Part model, mm, in its own coordinate system. Give positions to 0.01 mm unless a question says otherwise; leave off trailing zeros. Write each loop counter-clockwise with the first axis right and the second up, starting at its lowest first coordinate (ties: lowest second). Pieces come first, ordered by that corner, then holes.
from build123d import *

# Parameters (mm, degrees)
SKETCH_1_R      = 2
SKETCH_1_R_2    = 3.5
SKETCH_1_R_3    = 1
EXTRUDE_2_DEPTH = 0.5


with BuildPart() as part:
    # Эскиз1 → Бобышка-Вытянуть2 (new body)
    with BuildSketch(Plane(origin=(0, 0, 0), x_dir=(1, 0, 0), z_dir=(0, 1, 0))):
        with BuildLine():
            Line((-100, 38.5), (100, 38.5))
            ThreePointArc((100, 38.5), (100.707106781, 38.207106781), (101, 37.5))
            Line((101, 37.5), (101, -37.5))
            ThreePointArc((101, -37.5), (100.707106781, -38.207106781), (100, -38.5))
            Line((100, -38.5), (-100, -38.5))
            ThreePointArc((-100, -38.5), (-100.707106781, -38.207106781), (-101, -37.5))
            Line((-101, -37.5), (-101, 37.5))
            ThreePointArc((-101, 37.5), (-100.707106781, 38.207106781), (-100, 38.5))
        make_face()
        with Locations(Location((-88, 29, 0), (0, 0, 270))):
            Circle(SKETCH_1_R, mode=Mode.SUBTRACT)
        with Locations(Location((88, 29, 0), (0, 0, 270))):
            Circle(SKETCH_1_R, mode=Mode.SUBTRACT)
        with Locations(Location((88, -29, 0), (0, 0, 270))):
            Circle(SKETCH_1_R, mode=Mode.SUBTRACT)
        with Locations(Location((-88, -29, 0), (0, 0, 270))):
            Circle(SKETCH_1_R, mode=Mode.SUBTRACT)
        with Locations(Location((92, -10, 0), (0, 0, 270))):
            Circle(SKETCH_1_R_2, mode=Mode.SUBTRACT)
        with Locations(Location((0, 3, 0), (0, 0, 270))):
            Circle(SKETCH_1_R_3, mode=Mode.SUBTRACT)
        with Locations(Location((0, 7, 0), (0, 0, 270))):
            Circle(SKETCH_1_R_3, mode=Mode.SUBTRACT)
        with Locations(Location((0, 11, 0), (0, 0, 270))):
            Circle(SKETCH_1_R_3, mode=Mode.SUBTRACT)
        with Locations(Location((0, 15, 0), (0, 0, 270))):
            Circle(SKETCH_1_R_3, mode=Mode.SUBTRACT)
        with Locations(Location((0, 19, 0), (0, 0, 270))):
            Circle(SKETCH_1_R_3, mode=Mode.SUBTRACT)
        with Locations(Location((2.598076211, 1.5, 0), (0, 0, 270))):
            Circle(SKETCH_1_R_3, mode=Mode.SUBTRACT)
        with Locations(Location((6.062177826, 3.5, 0), (0, 0, 270))):
            Circle(SKETCH_1_R_3, mode=Mode.SUBTRACT)
        with Locations(Location((9.526279442, 5.5, 0), (0, 0, 270))):
            Circle(SKETCH_1_R_3, mode=Mode.SUBTRACT)
        with Locations(Location((12.990381057, 7.5, 0), (0, 0, 270))):
            Circle(SKETCH_1_R_3, mode=Mode.SUBTRACT)
        with Locations(Location((16.454482672, 9.5, 0), (0, 0, 270))):
            Circle(SKETCH_1_R_3, mode=Mode.SUBTRACT)
        with Locations(Location((2.598076211, -1.5, 0), (0, 0, 270))):
            Circle(SKETCH_1_R_3, mode=Mode.SUBTRACT)
        with Locations(Location((6.062177826, -3.5, 0), (0, 0, 270))):
            Circle(SKETCH_1_R_3, mode=Mode.SUBTRACT)
        with Locations(Location((9.526279442, -5.5, 0), (0, 0, 270))):
            Circle(SKETCH_1_R_3, mode=Mode.SUBTRACT)
        with Locations(Location((12.990381057, -7.5, 0), (0, 0, 270))):
            Circle(SKETCH_1_R_3, mode=Mode.SUBTRACT)
        with Locations(Location((16.454482672, -9.5, 0), (0, 0, 270))):
            Circle(SKETCH_1_R_3, mode=Mode.SUBTRACT)
        with Locations(Location((0, -3, 0), (0, 0, 270))):
            Circle(SKETCH_1_R_3, mode=Mode.SUBTRACT)
        with Locations(Location((0, -7, 0), (0, 0, 270))):
            Circle(SKETCH_1_R_3, mode=Mode.SUBTRACT)
        with Locations(Location((0, -11, 0), (0, 0, 270))):
            Circle(SKETCH_1_R_3, mode=Mode.SUBTRACT)
        with Locations(Location((0, -15, 0), (0, 0, 270))):
            Circle(SKETCH_1_R_3, mode=Mode.SUBTRACT)
        with Locations(Location((0, -19, 0), (0, 0, 270))):
            Circle(SKETCH_1_R_3, mode=Mode.SUBTRACT)
        with Locations(Location((-2.598076211, -1.5, 0), (0, 0, 270))):
            Circle(SKETCH_1_R_3, mode=Mode.SUBTRACT)
        with Locations(Location((-6.062177826, -3.5, 0), (0, 0, 270))):
            Circle(SKETCH_1_R_3, mode=Mode.SUBTRACT)
        with Locations(Location((-9.526279442, -5.5, 0), (0, 0, 270))):
            Circle(SKETCH_1_R_3, mode=Mode.SUBTRACT)
        with Locations(Location((-12.990381057, -7.5, 0), (0, 0, 270))):
            Circle(SKETCH_1_R_3, mode=Mode.SUBTRACT)
        with Locations(Location((-16.454482672, -9.5, 0), (0, 0, 270))):
            Circle(SKETCH_1_R_3, mode=Mode.SUBTRACT)
        with Locations(Location((-2.598076211, 1.5, 0), (0, 0, 270))):
            Circle(SKETCH_1_R_3, mode=Mode.SUBTRACT)
        with Locations(Location((-6.062177826, 3.5, 0), (0, 0, 270))):
            Circle(SKETCH_1_R_3, mode=Mode.SUBTRACT)
        with Locations(Location((-9.526279442, 5.5, 0), (0, 0, 270))):
            Circle(SKETCH_1_R_3, mode=Mode.SUBTRACT)
        with Locations(Location((-12.990381057, 7.5, 0), (0, 0, 270))):
            Circle(SKETCH_1_R_3, mode=Mode.SUBTRACT)
        with Locations(Location((-16.454482672, 9.5, 0), (0, 0, 270))):
            Circle(SKETCH_1_R_3, mode=Mode.SUBTRACT)
        with BuildLine():
            Line((-50.5, -31), (-50.5, -26))
            ThreePointArc((-50.5, -26), (-50, -25.5), (-49.5, -26))
            Line((-49.5, -26), (-49.5, -31))
            ThreePointArc((-49.5, -31), (-50, -31.5), (-50.5, -31))
        make_face(mode=Mode.SUBTRACT)
        with BuildLine():
            Line((-50.5, -17), (-50.5, -12))
            ThreePointArc((-50.5, -12), (-50, -11.5), (-49.5, -12))
            Line((-49.5, -12), (-49.5, -17))
            ThreePointArc((-49.5, -17), (-50, -17.5), (-50.5, -17))
        make_face(mode=Mode.SUBTRACT)
        with BuildLine():
            Line((49.5, -31), (49.5, -26))
            ThreePointArc((49.5, -26), (50, -25.5), (50.5, -26))
            Line((50.5, -26), (50.5, -31))
            ThreePointArc((50.5, -31), (50, -31.5), (49.5, -31))
        make_face(mode=Mode.SUBTRACT)
        with BuildLine():
            Line((49.5, -17), (49.5, -12))
            ThreePointArc((49.5, -12), (50, -11.5), (50.5, -12))
            Line((50.5, -12), (50.5, -17))
            ThreePointArc((50.5, -17), (50, -17.5), (49.5, -17))
        make_face(mode=Mode.SUBTRACT)
        with BuildLine():
            Line((49.5, -3), (49.5, 2))
            ThreePointArc((49.5, 2), (50, 2.5), (50.5, 2))
            Line((50.5, 2), (50.5, -3))
            ThreePointArc((50.5, -3), (50, -3.5), (49.5, -3))
        make_face(mode=Mode.SUBTRACT)
        with BuildLine():
            Line((49.5, 11), (49.5, 16))
            ThreePointArc((49.5, 16), (50, 16.5), (50.5, 16))
            Line((50.5, 16), (50.5, 11))
            ThreePointArc((50.5, 11), (50, 10.5), (49.5, 11))
        make_face(mode=Mode.SUBTRACT)
        with BuildLine():
            Line((49.5, 25), (49.5, 30))
            ThreePointArc((49.5, 30), (50, 30.5), (50.5, 30))
            Line((50.5, 30), (50.5, 25))
            ThreePointArc((50.5, 25), (50, 24.5), (49.5, 25))
        make_face(mode=Mode.SUBTRACT)
        with BuildLine():
            Line((-50.5, -3), (-50.5, 2))
            ThreePointArc((-50.5, 2), (-50, 2.5), (-49.5, 2))
            Line((-49.5, 2), (-49.5, -3))
            ThreePointArc((-49.5, -3), (-50, -3.5), (-50.5, -3))
        make_face(mode=Mode.SUBTRACT)
        with BuildLine():
            Line((-50.5, 11), (-50.5, 16))
            ThreePointArc((-50.5, 16), (-50, 16.5), (-49.5, 16))
            Line((-49.5, 16), (-49.5, 11))
            ThreePointArc((-49.5, 11), (-50, 10.5), (-50.5, 11))
        make_face(mode=Mode.SUBTRACT)
        with BuildLine():
            Line((-50.5, 25), (-50.5, 30))
            ThreePointArc((-50.5, 30), (-50, 30.5), (-49.5, 30))
            Line((-49.5, 30), (-49.5, 25))
            ThreePointArc((-49.5, 25), (-50, 24.5), (-50.5, 25))
        make_face(mode=Mode.SUBTRACT)
    extrude(amount=EXTRUDE_2_DEPTH)


solid = part.part
1) Saw through at B-B (x = -88). Write the cut outline in (y, z), and give its area (3 significant figures).
Check result:
outline: (0, -38.5) - (0.5, -38.5) - (0.5, -31) - (0, -31) - close; (0, -27) - (0.5, -27) - (0.5, 27) - (0, 27) - close; (0, 31) - (0.5, 31) - (0.5, 38.5) - (0, 38.5) - close
area: 34.5 mm2
2) Mould opens along Z. For faces 1 (the flat face through (1, 0.5, -1)), 2 (the cylindrical face through (-86.314, 0.246, -27.925)) say: +Z half, -Z half, draft (parallel to the pull), parting line (faces both ways), or undercut.
Check result:
face 1: draft
face 2: undercut
3) Drill centre lines: L1, parallel to X at y = 0.35, z = 1.5; L2, parallel to X at y = 0.2, z = 15; L3, parallel to X at y = 0.3, z = -3.5. Where is each one in solid material? Low to high.
Check result:
L1: x = -101 to -50.5, -49.5 to -3.6, -1.6 to 1.6, 3.6 to 49.5, 50.5 to 101
L2: x = -101 to -50.5, -49.5 to -1, 1 to 49.5, 50.5 to 101
L3: x = -101 to -7.06, -5.06 to -0.87, 0.87 to 5.06, 7.06 to 101
4) Saw through at C-C (y = 0.35). State how many separate pieces and enclosed holes the cut face has, and give its area (3 significant figures).
Check result:
separate pieces: 1
enclosed holes: 45
area: 15,300 mm2
5) Saw through at A-A (z = 29). Write the cut outline in (x, y).
Check result:
outline: (-101, 0) - (-90, 0) - (-90, 0.5) - (-101, 0.5) - close; (-86, 0) - (-50.5, 0) - (-50.5, 0.5) - (-86, 0.5) - close; (-49.5, 0) - (49.5, 0) - (49.5, 0.5) - (-49.5, 0.5) - close; (50.5, 0) - (86, 0) - (86, 0.5) - (50.5, 0.5) - close; (90, 0) - (101, 0) - (101, 0.5) - (90, 0.5) - close
